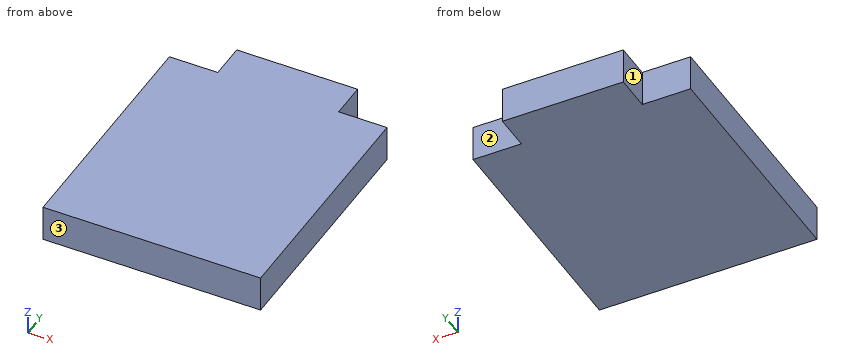
Autodesk Inventor part; units mm, degrees
ref_plane "YZ Plane" through (0, 0, 0) normal (1, 0, 0) x (0, 1, 0)
ref_plane "XZ Plane" through (0, 0, 0) normal (0, 1, 0) x (-1, 0, 0)
ref_plane "XY Plane" through (0, 0, 0) normal (0, 0, 1) x (1, 0, 0)
sketch "Sketch1" plane through (0, 0, 0) normal (0, 0, 1) x (1, 0, 0)
  line L0 (9, 0) -> (9, -20)
  line L1 (9, -20) -> (-9, -20)
  line L2 (-9, -20) -> (-9, 0)
  line L3 (-5, 0) -> (-5, 3)
  line L4 (-5, 3) -> (5, 3)
  line L5 (5, 3) -> (5, 0)
  line L6 (-9, 0) -> (-5, 0)
  line L7 (5, 0) -> (9, 0)
  line L8 (0, 0) -> (0, 3) construction
  line L9 (0, 0) -> (-9, 0) construction
  dimension "d0" = 18
  dimension "d1" = 4
  dimension "d2" = 3
  dimension "d3" = 20
extrude "Extrusion1" add sketch "Sketch1" along normal blind 3
properties part number "electromagnet_mnt_p2"
For this review, take the finished solid that the model builds, in its own axes (mm). Face numbers are marked on the shaded views. A direction names the side the tool comes from. Round coordinates to 2 decimals unless told otherwise and drop trailing zeros. Write each loop counter-clockwise with the first axis right and the second up, starting at its lowest first coordinate (ties: lowest second). Pieces come first, ordered by that corner, then holes. Notation, with made-up numbers: (60.25, 45) -> (106.25, 45) arc R13 cw to (106.25, 70) -> close; hole circle Ø7 at (54, 45). An arc over 180 degrees is marked (long way). Put each result on its own line as item: value.
Q1. Consider section A-A on z = 0.65. State the section outline as (x, y) points, and give its area (3 significant figures).
Determined:
outline: (-9, -20) -> (9, -20) -> (9, 0) -> (5, 0) -> (5, 3) -> (-5, 3) -> (-5, 0) -> (-9, 0) -> close
area: 390 mm^2
Q2. To check wall thickness, follow L1, parallel to X at y = 0.5, z = 1.8; L2, parallel to Y at x = 7, z = 0.35. State the ranges of each line that lie inside material, in increasing order. Write a range as [from, to].
Determined:
L1: x = [-5, 5]
L2: y = [-20, 0]
Q3. Consider section B-B on x = 7.5. State the section outline as (y, z) points, and give its area (3 significant figures).
Determined:
outline: (-20, 0) -> (0, 0) -> (0, 3) -> (-20, 3) -> close
area: 60.0 mm^2
Q4. Clearance check with a flat-ended pin moving along its axis: pin 1 Ø1.5 at (x, z) = (7, 1) entering from +Y. State where the tip first meets the part, or that it passes through.
Determined:
pin 1: stops at y = 0
Q5. Machinability: for the marked faces 1, 2 and 3, which of the approach directions +Z, -Z, +X, -X, +Y, -Y give a long, thin tool a straight path to every point of the face, cutting with its end or side? Answer none if there is none.
Determined:
face 1: +Z, -Z, -X, +Y
face 2: +Z, -Z, +X, +Y
face 3: +Z, -Z, +X, -X, -Y
Q6. Consider section C-C on y = 0.5. State the section outline as (x, z) points.
Determined:
outline: (-5, 0) -> (5, 0) -> (5, 3) -> (-5, 3) -> close
